Geometry: final body of the model. Coordinates: model frame, mm. A direction names the side the tool comes from. Give positions to 0.01 mm unless a question says otherwise; leave off trailing zeros. Write each loop counter-clockwise with the first axis right and the second up, starting at its lowest first coordinate (ties: lowest second). Pieces come first, ordered by that corner, then holes. Notation, with made-up numbers: (-25, -27) -> (-1, -27) arc R18 ccw to (-1, -11) -> close; hole circle Ø9 at (-23, 14.5). An arc over 180 degrees is marked (long way). Answer in a Markdown table with one row per item. Add a question column.
Item 1: First-contact query: P1, Ø1.5, axis at y = 9.5, z = -6.5, coming from the -X side; P2, Ø5, axis at x = -2.5, y = 2.5, coming from the +Z side; P3, Ø5, axis at x = -2.5, y = 6.5, coming from the +Z side. Flat tips, straight axial feed; report the tip coordinate or a pass-through.
Item 2: Section query B-B on y = 8.25. Output: boundary loops of the cut face in (x, z).
Item 3: Section query D-D on y = 9.75. Output: boundary loops of the cut face in (x, z), plus the area to 3 significant figures.
Item 4: Draft query along Z for faces 4 (the flat face through (3.3, 12, -0.1)), 5 (the cylindrical face through (0.77, 7.62, 2.43)), 6 (the flat face through (14, 1, -1.2)), 7 (the conical face through (-8.254, 0.28, -0.348)). Return one class per face: +Z half, -Z half, draft (parallel to the pull), parting line (faces both ways), or undercut.
Item 5: Section query C-C on y = 1. Output: boundary loops of the cut face in (x, z).
Item 6: Access query for faces 1 (the flat face through (14, 2.4, 0)), 2 (the flat face through (0, 4, 0)), 3 (the flat face through (3, 0, 0)). Directions: +Z, -Z, +X, -X, +Y, -Y. A direction counts if a zero-diameter tool reaches every point of the face in a straight line with its end or side. Return the directions, or none.
Item 7: Material intervals for probe 1 along Z at (x, y) = (0.25, 4.75); probe 2 along Z at (x, y) = (18, 1.25); probe 3 along Y at (x, z) = (18.25, 1), sorted ascending. Write a range as from..to.
Item 8: Section query A-A on x = 0. Output: boundary loops of the cut face in (y, z), plus the area to 3 significant figures.
```python
from build123d import *

# Parameters (mm, degrees)
SKETCH_1_R          = 9.1
EXTRUDE_1_DEPTH     = 12
EXTRUDE_1_TAPER     = 2.5
SKETCH_2_R          = 2.55
CUT_EXTRUDE_1_DEPTH = 8
SKETCH_3_W          = 13
SKETCH_3_H          = 2.4
EXTRUDE_2_DEPTH     = 2.4
CHAMFER_1_SIZE      = 0.5
CHAMFER_1_SIZE2     = 0.866025404
CHAMFER_2_SIZE      = 1
CHAMFER_2_SIZE2     = 1.611810972
CHAMFER_3_SIZE      = 1.87553439
CHAMFER_3_SIZE_2    = 1


with BuildPart() as part:
    # 草图1 → 凸台-拉伸1 (new body)
    with BuildSketch(Plane(origin=(0, 0, 0), x_dir=(1, 0, 0), z_dir=(0, 1, 0))):
        Circle(SKETCH_1_R)
    extrude(amount=EXTRUDE_1_DEPTH, taper=EXTRUDE_1_TAPER)

    # 草图2 → 切除-拉伸1 (cut)
    with BuildSketch(Plane(origin=(0, 12, 0), x_dir=(1, 0, 0), z_dir=(0, 1, 0))):
        with Locations(Location((0, 0, 0), (0, 0, 270))):
            Circle(SKETCH_2_R)
    extrude(amount=-CUT_EXTRUDE_1_DEPTH, mode=Mode.SUBTRACT)

    # 草图3 → 凸台-拉伸2 (add)
    with BuildSketch(Plane.XZ):
        with Locations((13.5, 0)):
            Rectangle(SKETCH_3_W, SKETCH_3_H)
    extrude(amount=-EXTRUDE_2_DEPTH)

    # 倒角1
    chamfer_1_edges = [part.edges().sort_by_distance(p)[0] for p in [
        (0, 12, -2.55),
    ]]
    chamfer_1_side = [part.faces().sort_by_distance(p)[0] for p in [
        (-8.333500832, 12, 0),
    ]]
    chamfer(chamfer_1_edges, length=CHAMFER_1_SIZE, length2=CHAMFER_1_SIZE2, reference=chamfer_1_side[0])

    # 倒角2
    chamfer_2_edges = [part.edges().sort_by_distance(p)[0] for p in [
        (-9.1, 0, 0),
    ]]
    chamfer_2_side = [part.faces().sort_by_distance(p)[0] for p in [
        (1.331118316, 0, 0),
    ]]
    chamfer(chamfer_2_edges, length=CHAMFER_2_SIZE, length2=CHAMFER_2_SIZE2, reference=chamfer_2_side[0])

    # 倒角3
    # the kernel refuses this chamfer: 1.87553439, 1 mm, written as the material it takes off along each edge
    with BuildSketch(Plane(origin=(0, 12, 0), x_dir=(1, 0, 0), z_dir=(0, 0, -1))) as chamfer_3_piece_1:
        Polygon((8.576068685 + CHAMFER_3_SIZE * 0.0436193873717, CHAMFER_3_SIZE * 0.999048221729), (8.576068685 - CHAMFER_3_SIZE_2, 0), (8.576068685, 0), align=None)
    revolve(axis=Axis((0, 12, 0), (0, -1, 0)), mode=Mode.SUBTRACT)


solid = part.part
```
Findings below:
| question | item | result |
|---|---|---|
| 1 | P1 | stops at x = -6.51 |
| 1 | P2 | stops at z = 9.03 |
| 1 | P3 | stops at z = 8.87 |
| 2 | outline | circle Ø17.48 at (0, 0); hole circle Ø5.1 at (0, 0) |
| 3 | outline | circle Ø17.35 at (0, 0); hole circle Ø5.1 at (0, 0) |
| 3 | area | 216 mm^2 |
| 4 | face 4 | draft |
| 4 | face 5 | undercut |
| 4 | face 6 | -Z half |
| 4 | face 7 | parting line |
| 5 | outline | (8.59, -1.2) -> (20, -1.2) -> (20, 1.2) -> (8.59, 1.2) arc R8.68 ccw (long way) to start |
| 6 | face 1 | +Z, -Z, +X, +Y |
| 6 | face 2 | +Y |
| 6 | face 3 | +Z, -Z, +X, -X, -Y |
| 7 | probe 1 | z = -8.89..-2.54, 2.54..8.89 |
| 7 | probe 2 | z = -1.2..1.2 |
| 7 | probe 3 | y = 0..2.4 |
| 8 | outline | (0, -8.1) -> (1.61, -9.03) -> (10.13, -8.66) -> (12, -7.58) -> (12, -3.05) -> (11.13, -2.55) -> (4, -2.55) -> (4, 2.55) -> (11.13, 2.55) -> (12, 3.05) -> (12, 7.58) -> (10.13, 8.66) -> (1.61, 9.03) -> (0, 8.1) -> close |
| 8 | area | 167 mm^2 |
